from build123d import *

# Parameters (mm, degrees)
SKETCH2_R           = 37.5
BOSS_EXTRUDE1_DEPTH = 30
SKETCH4_R           = 2.5
CUT_EXTRUDE2_DEPTH  = 25
SKETCH5_W           = 14
SKETCH5_H           = 42
CUT_EXTRUDE3_DEPTH  = 57.5
SKETCH6_R           = 20.385544883
CUT_EXTRUDE4_DEPTH  = 57.5


with BuildPart() as part:
    # Sketch2 → Boss-Extrude1 (new body)
    with BuildSketch(Plane(origin=(0, 0, 0), x_dir=(1, 0, 0), z_dir=(0, 1, 0))):
        with Locations(Location((0, 0, 0), (0, 0, 270))):
            Circle(SKETCH2_R)
    extrude(amount=BOSS_EXTRUDE1_DEPTH)

    # Sketch4 → Cut-Extrude2 (cut)
    with BuildSketch(Plane(origin=(0, 30, 0), x_dir=(1, 0, 0), z_dir=(0, 1, 0))):
        with Locations(Location((22, 24, 0), (0, 0, 270))):
            Circle(SKETCH4_R)
        with Locations(Location((24, -22, 0), (0, 0, 270))):
            Circle(SKETCH4_R)
        with Locations(Location((-22, -24, 0), (0, 0, 270))):
            Circle(SKETCH4_R)
        with Locations(Location((-24, 22, 0), (0, 0, 270))):
            Circle(SKETCH4_R)
    extrude(amount=-CUT_EXTRUDE2_DEPTH, mode=Mode.SUBTRACT)

    # Sketch5 → Cut-Extrude3 (cut, symmetric)
    with BuildSketch(Plane.XY):
        Rectangle(SKETCH5_W, SKETCH5_H)
    extrude(amount=CUT_EXTRUDE3_DEPTH, both=True, mode=Mode.SUBTRACT)

    # Sketch6 → Cut-Extrude4 (cut, symmetric)
    with BuildSketch(Plane(origin=(0, 30, 0), x_dir=(1, 0, 0), z_dir=(0, 1, 0))):
        with Locations(Location((0, 0, 0), (0, 0, 270))):
            Circle(SKETCH6_R)
    extrude(amount=CUT_EXTRUDE4_DEPTH, both=True, mode=Mode.SUBTRACT)


solid = part.part
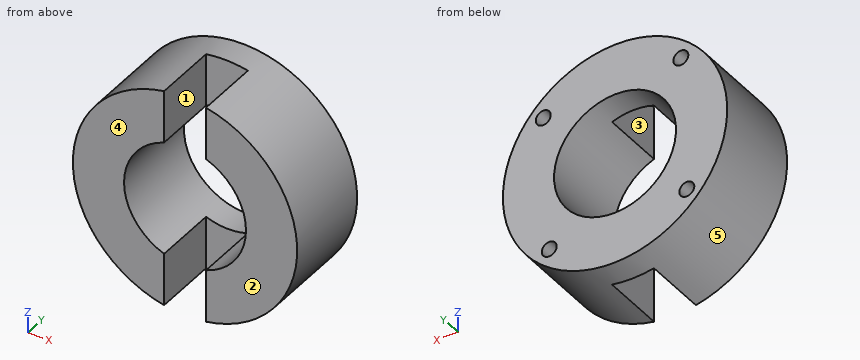
For this review, take the finished solid that the model builds, in its own axes (mm). Face numbers are marked on the shaded views. A direction names the side the tool comes from. Give positions to 0.01 mm unless a question says otherwise; leave off trailing zeros. Order: outer loops, then holes, each group sorted by start corner. A loop starts at its lowest first (then second) coordinate and runs counter-clockwise, first axis right, second up. Notation, with made-up numbers: M 29.25,-5.5 L 46.25,-5.5 A20 ccw 46.25,10.5 Z; hole C 4.25,84.5 d6. An arc over 180 degrees is marked long. Answer in a Markdown table with one row per item. Add a question column.
(1) Mouldability with a two-part tool opening along X and no side actions: class the marked faces 3, 4 and 5 as +X half, -X half, draft (parallel to the pull), parting line (faces both ways), or undercut.
(2) Consider section B-B on z = -14. State the section outline as (x, y) points, and give its area (3 significant figures).
(3) For the marked faces 1 and 2, list the 3-axis set-ups (+Z, -Z, +X, -X, +Y, -Y) from which the entire face can be reached by the end or side of a thin tool; tool diameter is ignored.
(4) Consider section D-D on y = 28. State the section outline as (x, z) points, and give its area (3 significant figures).
(5) Wall thickness on probe 1 along Z at (x, y) = (7, 28.75); probe 2 along Z at (x, y) = (-23.5, 17.5); probe 3 along X at (y, z) = (22.5, -24): over which ranges is each line inside the solid? List them lowest first. Write a range as [from, to].
(6) Consider section A-A on y = 15.25. State the section outline as (x, z) points.
(7) Consider section C-C on x = 14. State the section outline as (y, z) points.
(8) For pin 1 (2 mm diameter, centred on x = -6.5, y = 8, fed in from -Z); pin 2 (4 mm diameter, centred on x = -24, z = -22, fed in from +Y); pin 3 (1 mm diameter, centred on x = -14.5, y = 13, fed in from +Z); pin 4 (2 mm diameter, centred on x = 6, z = -17, fed in from +Y), all flat-tipped, find the tip position at first contact; note any pin that passes through.
Evaluation:
| question | item | result |
|---|---|---|
| 1 | face 3 | undercut |
| 1 | face 4 | draft |
| 1 | face 5 | parting line |
| 2 | outline | M -34.79,0 L -14.82,0 L -14.82,30 L -34.79,30 Z; M 14.82,0 L 34.79,0 L 34.79,30 L 14.82,30 Z |
| 2 | area | 1,200 mm^2 |
| 3 | face 1 | +Z, -Z, -Y |
| 3 | face 2 | +Z, -Z, +X, -X, -Y |
| 4 | outline | C 0,0 d75; hole C -24,-22 d5; hole C -22,24 d5; hole C 0,0 d40.77; hole C 22,-24 d5; hole C 24,22 d5 |
| 4 | area | 3,030 mm^2 |
| 5 | probe 1 | z = [-36.84, -19.15], [19.15, 36.84] |
| 5 | probe 2 | z = [-29.22, -24.45], [-19.55, 22], [26, 29.22] |
| 5 | probe 3 | x = [-28.81, -25.5], [-22.5, 19.5], [24.5, 28.81] |
| 6 | outline | M -7,-36.84 L -7,-19.15 A20.39 cw -7,19.15 L -7,36.84 A37.5 ccw Z; M 7,-36.84 A37.5 ccw 7,36.84 L 7,19.15 A20.39 cw 7,-19.15 Z; hole C -24,-22 d5; hole C -22,24 d5; hole C 22,-24 d5; hole C 24,22 d5 |
| 7 | outline | M 0,-34.79 L 30,-34.79 L 30,-14.82 L 0,-14.82 Z; M 0,14.82 L 30,14.82 L 30,34.79 L 0,34.79 Z |
| 8 | pin 1 | stops at z = -36.84 |
| 8 | pin 2 | stops at y = 5 |
| 8 | pin 3 | stops at z = 34.79 |
| 8 | pin 4 | passes through |
